Build history of the part. All positions in model axes, mm. A direction names the side the tool comes from. Give positions to 0.01 mm unless a question says otherwise; leave off trailing zeros. Write each loop counter-clockwise with the first axis right and the second up, starting at its lowest first coordinate (ties: lowest second). Pieces come first, ordered by that corner, then holes. Notation, with made-up numbers: (20.25, 49) -> (64.25, 49) arc R28 ccw to (64.25, 81) -> close; hole circle Ø8 at (-3.75, -16.75). An arc over 180 degrees is marked (long way). Put each result on its own line as item: value. Start each with the question number.
Item 1: Slice it at A-A, the plane x = -14. List the corners of the cut face in (y, z).
Item 2: Slice it at B-B, the plane z = -47. List the corners of the cut face in (x, y), plus the area to 4 significant figures.
Item 3: Slice it at C-C, the plane y = 37. List the corners of the cut face in (x, z).
Item 4: Tool access for faces 1 (the flat face through (0, 39, -64)), 2 (the flat face through (0, 0, -63)), 3 (the flat face through (0, 19, -62.75)), 4 (the flat face through (-22.75, 20, 1)), 5 (the flat face through (-22, 44, 4)): list every direction of +Z, -Z, +X, -X, +Y, -Y with a clear straight run to the whole face (end or side of a thin tool).
Item 5: Flat gauge pins, fed straight in: pin 1 Ø12 at (x, z) = (-15.5, 17.5) entering from -Y; pin 2 Ø1.6 at (x, y) = (-21.5, -1) entering from +Z; pin 3 Ø1 at (x, y) = (16, 10.5) entering from +Z. Where does each tip first touch, or does it go through?
Item 6: Drill centre lines: line 1 along X through (y, z) = (36, -3.5); line 2 along Z through (x, y) = (19.5, 6.5). Where is each one in solid material? Low to high.
```python
from build123d import *

# Parameters (mm, degrees)
BOSS_EXTRUDE1_DEPTH = 39
SKETCH2_W           = 1.5
SKETCH2_H           = 92.5
BOSS_EXTRUDE2_DEPTH = 5
SKETCH3_W           = 1.5
SKETCH3_H           = 8
BOSS_EXTRUDE3_DEPTH = 2.5
SKETCH4_W           = 45.5
SKETCH4_H           = 5
BOSS_EXTRUDE5_DEPTH = 1.5


with BuildPart() as part:
    # Sketch1 → Boss-Extrude1 (new body)
    with BuildSketch(Plane(origin=(0, 0, 0), x_dir=(1, 0, 0), z_dir=(0, 1, 0))):
        Polygon((22.75, 64.25), (22.75, -64.25), (21.25, -64.25), (21.25, 62.75), (-21.25, 62.75), (-21.25, -64.25), (-22.75, -64.25), (-22.75, 64.25), align=None)
    extrude(amount=BOSS_EXTRUDE1_DEPTH)

    # Sketch2 → Boss-Extrude2 (add)
    with BuildSketch(Plane(origin=(0, 39, 0), x_dir=(1, 0, 0), z_dir=(0, 1, 0))):
        with Locations((-22, -18)):
            Rectangle(SKETCH2_W, SKETCH2_H)
        with Locations((22, -18)):
            Rectangle(SKETCH2_W, SKETCH2_H)
    extrude(amount=BOSS_EXTRUDE2_DEPTH)

    # Sketch3 → Boss-Extrude3 (add)
    with BuildSketch(Plane.XZ):
        with Locations((22, -47.75)):
            Rectangle(SKETCH3_W, SKETCH3_H)
        with Locations((-22, -47.75)):
            Rectangle(SKETCH3_W, SKETCH3_H)
        with Locations((22, 47.75)):
            Rectangle(SKETCH3_W, SKETCH3_H)
        with Locations((-22, 47.75)):
            Rectangle(SKETCH3_W, SKETCH3_H)
    extrude(amount=BOSS_EXTRUDE3_DEPTH)

    # Sketch4 → Boss-Extrude5 (add)
    with BuildSketch(Plane(origin=(0, 0, -28.25), x_dir=(-1, 0, 0), z_dir=(0, 0, -1))):
        with Locations((0, 41.5)):
            Rectangle(SKETCH4_W, SKETCH4_H)
    extrude(amount=-BOSS_EXTRUDE5_DEPTH)


solid = part.part
```
Values follow:
1. outline: (0, -64.25) -> (39, -64.25) -> (39, -62.75) -> (0, -62.75) -> close; (39, -28.25) -> (44, -28.25) -> (44, -26.75) -> (39, -26.75) -> close
2. outline: (-22.75, -2.5) -> (-21.25, -2.5) -> (-21.25, 39) -> (-22.75, 39) -> close; (21.25, -2.5) -> (22.75, -2.5) -> (22.75, 39) -> (21.25, 39) -> close
2. area: 124.5 mm2
3. outline: (-22.75, -64.25) -> (22.75, -64.25) -> (22.75, 64.25) -> (21.25, 64.25) -> (21.25, -62.75) -> (-21.25, -62.75) -> (-21.25, 64.25) -> (-22.75, 64.25) -> close
4. face 1: -Z, +X, -X, +Y
4. face 2: -Z, +X, -X, -Y
4. face 3: +Z, +Y, -Y
4. face 4: +Z, -Z, -X, +Y, -Y
4. face 5: +Z, -Z, +X, -X, +Y
5. pin 1: y = 0
5. pin 2: z = 51.75
5. pin 3: z = -62.75
6. line 1: -22.75 to -21.25, 21.25 to 22.75
6. line 2: -64.25 to -62.75
